The model under review builds one solid part; all positions refer to its coordinate system, in mm. Face numbers are marked on the shaded views. A direction names the side the tool comes from. Round coordinates to 2 decimals unless told otherwise and drop trailing zeros. Write each loop counter-clockwise with the first axis right and the second up, starting at its lowest first coordinate (ties: lowest second). Pieces come first, ordered by that corner, then holes. Notation, with made-up numbers: (67.5, -31.5) -> (113.5, -31.5) arc R21 ccw to (113.5, -26.5) -> close; hole circle Ø9 at (73.25, -18.75). An arc over 180 degrees is marked (long way). Return JSON: item names as keys, results as strings. Group by question number.
1. Take a section at A-A, the plane x = -5. Write out the cut boundary in (y, z).
2. Take a section at B-B, the plane z = 15. Write out the cut boundary in (x, y), then the cut area to 3 significant figures.
3. For line 1 along Z through (x, y) = (-15, -3); line 2 along X through (y, z) = (-4, 5); line 3 along Z through (x, y) = (-5, -3.25), list the stretches that pass through material, from the lowest coordinate up. Write a range as from..to.
4. Take a section at C-C, the plane y = -1.5. Write out the cut boundary in (x, z), then the cut area to 3 significant figures.
5. Mouldability with a two-part tool opening along Z and no side actions: class the marked faces 1, 2 and 3 as pulls with the +Z half, pulls with the -Z half, needs draft (parallel to the pull), parting line crosses it, or undercut.
6. Tool access review of the marked faces 4 and 5: name each direction out of +Z, -Z, +X, -X, +Y, -Y from which nothing blocks a thin tool from reaching the whole face with its end or side.
7. Clearance check with flat-ended pins moving along their axes: P1, Ø2.5, axis at x = -5, z = 15, coming from the +Y side; P2, Ø3, axis at y = -2.5, z = 15, coming from the -X side; P3, Ø5, axis at x = -14, y = -2.5, coming from the +Z side; P4, Ø4, axis at x = -15, z = 5, coming from the -Y side. State where each tip first meets the part, or that it passes through.
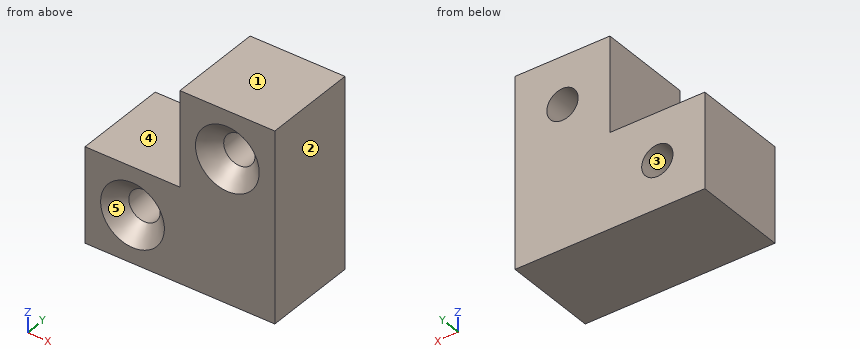
from build123d import *

# Parameters (mm, degrees)
F1_DEPTH       = 10
F3_D           = 3.3
F3_CSINK_D     = 6.72
F3_CSINK_ANGLE = 90


with BuildPart() as f1:
    # F0 (on Front) → F1 (new body)
    with BuildSketch(Plane.XZ):
        Polygon((0, 20), (-10, 20), (-10, 10), (-20, 10), (-20, 0), (0, 0), align=None)
    extrude(amount=F1_DEPTH)

    # F3 (through all)
    with Locations(Plane.XZ.offset(10)):
        with Locations((-5, 15), (-15, 5)):
            CounterSinkHole(F3_D / 2, F3_CSINK_D / 2, counter_sink_angle=F3_CSINK_ANGLE)


solid = f1.part
Output:
{
 "1": {"outline": "(-10, 0) -> (0, 0) -> (0, 13.35) -> (-8.29, 13.35) -> (-10, 11.64) -> close; (-10, 18.36) -> (-8.29, 16.65) -> (0, 16.65) -> (0, 20) -> (-10, 20) -> close"},
 "2": {"outline": "(-10, -10) -> (-8.36, -10) -> (-6.65, -8.29) -> (-6.65, 0) -> (-10, 0) -> close; (-3.35, -8.29) -> (-1.64, -10) -> (0, -10) -> (0, 0) -> (-3.35, 0) -> close", "area": "64.1 mm^2"},
 "3": {"line 1": "z = 0..3.35, 6.65..10", "line 2": "x = -20..-16.65, -13.35..0", "line 3": "z = 0..13.35, 16.65..20"},
 "4": {"outline": "(-20, 0) -> (0, 0) -> (0, 20) -> (-10, 20) -> (-10, 10) -> (-20, 10) -> close; hole circle Ø3.3 at (-15, 5); hole circle Ø3.3 at (-5, 15)", "area": "283 mm^2"},
 "5": {"face 1": "pulls with the +Z half", "face 2": "needs draft", "face 3": "undercut"},
 "6": {"face 4": "+Z, -X, +Y, -Y", "face 5": "-Y"},
 "7": {"P1": "passes through", "P2": "stops at x = -10", "P3": "stops at z = 10", "P4": "stops at y = -8.64"}
}
